```python
from build123d import *

# Parameters (mm, degrees)
F1_DEPTH      = 50
F2_DEPTH      = 3
F4_DEPTH      = 3
F5_W          = 30
F5_H          = 2
F6_DEPTH      = 25
F7_W          = 5
F7_H          = 12
F8_DEPTH      = 25
F9_SIZE       = 2
F11_DEPTH     = 7.5
F12_T1_DEPTH  = 26.3054072893
F13_T1_DEPTH  = 27.2441766919
F15_DEPTH     = 7.5
F16_T1_DEPTH  = 26.3054072893
F17_T1_DEPTH  = 27.2441766919
F18_R         = 5
F19_T4_DEPTH  = 100.8695078042
F19_T7_ANGLE  = 76.4615865705
F19_T11_DEPTH = 62.2556275763
F20_T4_DEPTH  = 100.8695078042
F20_T9_DEPTH  = 62.2556275763
F20_T12_ANGLE = 76.4615865705


# Not quite as in the source:
# - a fillet or chamfer that OpenCascade refuses, or shapes differently, is made with other operations: its cross-section is extruded or revolved along the edge and cut away or added


with BuildPart() as f1:
    # F0 (on Right) → F1 (new body)
    with BuildSketch(Plane.YZ):
        Polygon((28.4014230277, 3.870410641), (-56.2452584396, -38.2620337305), (-49.5127283639, -38.2620337305), (27.6224404883, 0.1315944002), (59.8385196924, -38.2620337305), (63.7547415604, -38.2620337305), align=None)
    extrude(amount=F1_DEPTH)

    # F0 (on Right) → F2 (join)
    with BuildSketch(Plane.YZ):
        Polygon((27.6224404883, 0.1315944002), (-49.5127283639, -38.2620337305), (59.8385196924, -38.2620337305), align=None)
    extrude(amount=F2_DEPTH)

    # F3 (on face) → F4 (join)
    with BuildSketch(Plane.YZ.offset(50)):
        Polygon((27.6224404883, 0.1315944002), (-49.5127283639, -38.2620337305), (59.8385196924, -38.2620337305), align=None)
    extrude(amount=-F4_DEPTH)

    # F5 (on face) → F6 (cut)
    with BuildSketch(Plane(origin=(0, 18.5724443931, 15.5841312403), x_dir=(-1, 0, 0), z_dir=(0, 0.7660444431, 0.6427876097))):
        with Locations((-25, -42.7911762555)):
            Rectangle(F5_W, F5_H)
    extrude(amount=-F6_DEPTH, mode=Mode.SUBTRACT)

    # F7 (on face) → F8 (cut)
    with BuildSketch(Plane(origin=(0, 4.0953498153, -8.2278105741), x_dir=(1, 0, 0), z_dir=(0, -0.4455977123, 0.8952333097))):
        with Locations((25, -51.4021035664)):
            Rectangle(F7_W, F7_H)
    extrude(amount=-F8_DEPTH, mode=Mode.SUBTRACT)

    # F9
    f9_edges = [f1.edges().sort_by_distance(p)[0] for p in [
        (25, -35.213332, -31.144584),
    ]]
    chamfer(f9_edges, length=F9_SIZE)

    # F10 (on face) → F11 (join)
    with BuildSketch(Plane(origin=(0, 0, 0), x_dir=(0, -1, 0), z_dir=(-1, 0, 0))):
        Polygon((56.2452584396, -38.2620337305), (54.2361967122, -37.2620337305), (-62.9156419292, -37.2620337305), (-63.7547415604, -38.2620337305), align=None)
    extrude(amount=F11_DEPTH)

    # F12: fillet of radius 5 on 1 edges, made by hand

    # F12_s2 → F12_t1 (cut)
    with BuildSketch(Plane(origin=(0, 36.3083524151, -43.2706094318), x_dir=(1, 0, 0), z_dir=(0, 0.6427876097, -0.7660444431))):
        with BuildLine():
            ThreePointArc((-7.5, -19.2446042914), (-6.0355339059, -22.7801381974), (-2.5, -24.2446042914))
            Line((-2.5, -24.2446042914), (-7.5, -24.2446042914))
            Line((-7.5, -24.2446042914), (-7.5, -19.2446042914))
        make_face()
    extrude(amount=F12_T1_DEPTH, mode=Mode.SUBTRACT)

    # F13: fillet of radius 5 on 1 edges, made by hand

    # F13_s2 → F13_t1 (cut)
    with BuildSketch(Plane(origin=(0, -71.5310246258, -35.6041945608), x_dir=(1, 0, 0), z_dir=(0, 0.8952333097, 0.4455977123))):
        with BuildLine():
            ThreePointArc((-2.5, 9.1906886005), (-6.0355339059, 10.6551546946), (-7.5, 14.1906886005))
            Line((-7.5, 14.1906886005), (-7.5, 9.1906886005))
            Line((-7.5, 9.1906886005), (-2.5, 9.1906886005))
        make_face()
    extrude(amount=F13_T1_DEPTH, mode=Mode.SUBTRACT)

    # F14 (on face) → F15 (join)
    with BuildSketch(Plane.YZ.offset(50)):
        Polygon((63.7547415604, -38.2620337305), (62.9156419292, -37.2620337305), (-54.2361967122, -37.2620337305), (-56.2452584396, -38.2620337305), align=None)
    extrude(amount=F15_DEPTH)

    # F16: fillet of radius 5 on 1 edges, made by hand

    # F16_s2 → F16_t1 (cut)
    with BuildSketch(Plane(origin=(0, 53.2171422884, -63.4217205098), x_dir=(1, 0, 0), z_dir=(0, -0.6427876097, 0.7660444431))):
        with BuildLine():
            ThreePointArc((52.5, 24.2446042914), (56.0355339059, 22.7801381974), (57.5, 19.2446042914))
            Line((57.5, 19.2446042914), (57.5, 24.2446042914))
            Line((57.5, 24.2446042914), (52.5, 24.2446042914))
        make_face()
    extrude(amount=F16_T1_DEPTH, mode=Mode.SUBTRACT)

    # F17: fillet of radius 5 on 1 edges, made by hand

    # F17_s2 → F17_t1 (cut)
    with BuildSketch(Plane(origin=(0, -47.1411301566, -23.4642517522), x_dir=(1, 0, 0), z_dir=(0, -0.8952333097, -0.4455977123))):
        with BuildLine():
            ThreePointArc((52.5, -9.1906886005), (56.0355339059, -10.6551546946), (57.5, -14.1906886005))
            Line((57.5, -14.1906886005), (57.5, -9.1906886005))
            Line((57.5, -9.1906886005), (52.5, -9.1906886005))
        make_face()
    extrude(amount=F17_T1_DEPTH, mode=Mode.SUBTRACT)

    # F18
    f18_edges = [f1.edges().sort_by_distance(p)[0] for p in [
        (25, 28.401423, 3.870411),
    ]]
    fillet(f18_edges, radius=F18_R)

    # F19: fillet of radius 5 on 3 edges, made by hand


with BuildPart() as f19_tool2:
    # F19_s3 → F19_t4 (new body)
    with BuildSketch(Plane(origin=(0, 20.7797804184, 10.3430273622), x_dir=(1, 0, 0), z_dir=(0, -0.8952333097, -0.4455977123))):
        with BuildLine():
            ThreePointArc((45, -9.1906886005), (48.5355339059, -10.6551546946), (50, -14.1906886005))
            Line((50, -14.1906886005), (50, -9.1906886005))
            Line((50, -9.1906886005), (45, -9.1906886005))
        make_face()
    extrude(amount=F19_T4_DEPTH)

    split(bisect_by=Plane.XY.offset(-37.2620337305), keep=Keep.TOP)


with BuildPart() as f1_1:
    add(f1.part)

    # F19_t1: cut F19_tool2
    add(f19_tool2.part, mode=Mode.SUBTRACT)

    # F19_s6 → F19_t7 (revolve, cut)
    with BuildSketch(Plane(origin=(0, 20.7797804184, 10.3430273622), x_dir=(1, 0, 0), z_dir=(0, -0.8952333097, -0.4455977123))):
        with BuildLine():
            ThreePointArc((45, -9.1906886005), (48.5355339059, -10.6551546946), (50, -14.1906886005))
            Line((50, -14.1906886005), (50, -9.1906886005))
            Line((50, -9.1906886005), (45, -9.1906886005))
        make_face()
    revolve(axis=Axis((50, 27.1031187954, -2.3609497603), (-1, 0, 0)), revolution_arc=F19_T7_ANGLE, mode=Mode.SUBTRACT)


with BuildPart() as f19_tool9:
    # F19_s10 → F19_t11 (new body)
    with BuildSketch(Plane(origin=(0, 52.3780426572, -62.4217205098), x_dir=(1, 0, 0), z_dir=(0, -0.6427876097, 0.7660444431))):
        with BuildLine():
            ThreePointArc((50, 19.2446042914), (48.5355339059, 22.7801381974), (45, 24.2446042914))
            Line((45, 24.2446042914), (50, 24.2446042914))
            Line((50, 24.2446042914), (50, 19.2446042914))
        make_face()
    extrude(amount=F19_T11_DEPTH)

    split(bisect_by=Plane.XY.offset(-37.2620337305), keep=Keep.TOP)


with BuildPart() as f1_2:
    add(f1_1.part)

    # F19_t8: cut F19_tool9
    add(f19_tool9.part, mode=Mode.SUBTRACT)

    # F20: fillet of radius 5 on 3 edges, made by hand


with BuildPart() as f20_tool2:
    # F20_s3 → F20_t4 (new body)
    with BuildSketch(Plane(origin=(0, 20.7797804184, 10.3430273622), x_dir=(1, 0, 0), z_dir=(0, -0.8952333097, -0.4455977123))):
        with BuildLine():
            ThreePointArc((5, -9.1906886005), (1.4644660941, -10.6551546946), (0, -14.1906886005))
            Line((0, -14.1906886005), (0, -9.1906886005))
            Line((0, -9.1906886005), (5, -9.1906886005))
        make_face()
    extrude(amount=F20_T4_DEPTH)

    split(bisect_by=Plane.XY.offset(-37.2620337305), keep=Keep.TOP)


with BuildPart() as f1_3:
    add(f1_2.part)

    # F20_t1: cut F20_tool2
    add(f20_tool2.part, mode=Mode.SUBTRACT)


with BuildPart() as f20_tool7:
    # F20_s8 → F20_t9 (new body)
    with BuildSketch(Plane(origin=(0, 52.3780426572, -62.4217205098), x_dir=(1, 0, 0), z_dir=(0, -0.6427876097, 0.7660444431))):
        with BuildLine():
            ThreePointArc((0, 19.2446042914), (1.4644660941, 22.7801381974), (5, 24.2446042914))
            Line((5, 24.2446042914), (0, 24.2446042914))
            Line((0, 24.2446042914), (0, 19.2446042914))
        make_face()
    extrude(amount=F20_T9_DEPTH)

    split(bisect_by=Plane.XY.offset(-37.2620337305), keep=Keep.TOP)


with BuildPart() as f1_4:
    add(f1_3.part)

    # F20_t6: cut F20_tool7
    add(f20_tool7.part, mode=Mode.SUBTRACT)

    # F20_s11 → F20_t12 (revolve, cut)
    with BuildSketch(Plane(origin=(0, 20.7797804184, 10.3430273622), x_dir=(1, 0, 0), z_dir=(0, -0.8952333097, -0.4455977123))):
        with BuildLine():
            ThreePointArc((0, -14.1906886005), (1.4644660941, -10.6551546946), (5, -9.1906886005))
            Line((5, -9.1906886005), (0, -9.1906886005))
            Line((0, -9.1906886005), (0, -14.1906886005))
        make_face()
    revolve(axis=Axis((0, 27.1031187954, -2.3609497603), (-1, 0, 0)), revolution_arc=F20_T12_ANGLE, mode=Mode.SUBTRACT)


solid = f1_4.part
```
The model under review builds one solid part; all positions refer to its coordinate system, in mm. A direction names the side the tool comes from. Round coordinates to 2 decimals unless told otherwise and drop trailing zeros. Order: outer loops, then holes, each group sorted by start corner. A loop starts at its lowest first (then second) coordinate and runs counter-clockwise, first axis right, second up. Notation, with made-up numbers: M 29.25,64 L 46.25,64 A6 ccw 46.25,75 Z; hole C -2.75,-37 d8. An arc over 180 degrees is marked long. Use a Markdown table: item, result.
1) Tool access review of faces 1 (the face through (40, 45, -18)), 2 (the face through (24.96, -34.78, -29.8)), 3 (the face through (3, 17, -23)), 4 (the face through (24.965, -46.634, -35.13)), 5 (the face through (0, 17, -23)): name each direction out of +Z, -Z, +X, -X, +Y, -Y from which nothing blocks a thin tool from reaching the whole face with its end or side.
Report:
| item | result |
|---|---|
| face 1 | none |
| face 2 | -Z, -Y |
| face 3 | -Z |
| face 4 | +Z |
| face 5 | +Z, -X, +Y, -Y |
2) Insertion check: pin 1 (6 mm diameter, centred on x = 10.5, y = -15.5, fed in from +Z); pin 2 (11.5 mm diameter, centred on y = 9.5, z = -17.5, fed in from -X); pin 3 (6.5 mm diameter, centred on y = -43.5, z = -31, fed in from +X). Each pin has a flat end and moves straight along its axis. Give the tip position at first contact, or say it passes through.
Report:
| item | result |
|---|---|
| pin 1 | z = -16.49 |
| pin 2 | x = 0 |
| pin 3 | x = 49.29 |
3) Wall thickness on line 1 along X through (y, z) = (-19.5, -28); line 2 along X through (y, z) = (-37, -33); line 3 along Y through (x, z) = (12.5, -1): over which ranges is each line inside the solid? List them lowest first. Write a range as [from, to].
Report:
| item | result |
|---|---|
| line 1 | [0, 3], [47, 50] |
| line 2 | [0.13, 3], [47, 49.87] |
| line 3 | [18.62, 25.35], [28.57, 32.49] |
4) Draft analysis for pull direction X (two halves, no side actions). For faces 6 (the face through (24.692, -11.485, -19.334)), 7 (the face through (1.426, 45.997, -19.438)), 8 (the face through (25.28, 28.169, 2.524)), state which applies: released by +X, released by -X, zero draft, split by the parting line, or undercut.
Report:
| item | result |
|---|---|
| face 6 | undercut |
| face 7 | released by -X |
| face 8 | zero draft |
5) Consider section A-A (x = 20). Write out the cut boundary in (y, z), then the cut area to 3 significant figures.
Report:
| item | result |
|---|---|
| outline | M -56.25,-38.26 L -49.51,-38.26 L 27.62,0.13 L 43.14,-18.36 L 45.44,-16.43 L 30.93,0.85 A5 ccw 24.88,2.12 Z; M 44.42,-19.89 L 59.84,-38.26 L 63.75,-38.26 L 46.72,-17.96 Z |
| area | 420 mm^2 |
